from build123d import *

# Parameters (mm, degrees)
SKETCH1_W                   = 800
SKETCH1_H                   = 50
BOSS_EXTRUDE1_DEPTH         = 30
SKETCH2_R                   = 40
BOSS_EXTRUDE2_DEPTH         = 370
FILLET5_RADIUS              = 25
FILLET5_LENGTH              = 30
FILLET6_R                   = 25
FILLET5_OF_MIRROR3_2_RADIUS = 25
FILLET5_OF_MIRROR3_2_LENGTH = 30
FILLET6_OF_MIRROR3_R        = 25
CUT_EXTRUDE3_DEPTH          = 589.680979382
CUT_EXTRUDE3_DEPTH_BACK     = 589.680979382
SKETCH5_R                   = 10
SKETCH6_R                   = 10
CUT_EXTRUDE4_DEPTH          = 589.680979382


with BuildPart() as part:
    # Sketch1 → Boss-Extrude1 (new body)
    with BuildSketch(Plane.XY):
        Rectangle(SKETCH1_W, SKETCH1_H)
    boss_extrude1 = extrude(amount=BOSS_EXTRUDE1_DEPTH)

    # Sketch2 → Boss-Extrude2 (add)
    with BuildSketch(Plane.XY.offset(30)):
        with Locations(Location((-360.056615351, 0, 0), (0, 0, 176.951220784))):
            Circle(SKETCH2_R)
    extrude(amount=BOSS_EXTRUDE2_DEPTH)

    # Fillet5: full round fillet: the end face becomes a half cylinder, R = half its width
    fillet5_face = Plane((400, 0, 15), x_dir=(0, 0, -1), z_dir=(1, 0, 0))  # on the end face: x along it, z out of the body
    fillet5_slab = fillet5_face.offset(-FILLET5_RADIUS / 2) * Box(FILLET5_LENGTH, 2 * FILLET5_RADIUS, FILLET5_RADIUS, mode=Mode.PRIVATE)  # the body's end, R deep
    fillet5_round = Plane((375, 0, 15), x_dir=(1, 0, 0), z_dir=(0, 0, -1)) * Cylinder(FILLET5_RADIUS, FILLET5_LENGTH, mode=Mode.PRIVATE)  # its axis R under the face
    add(fillet5_slab - fillet5_round, mode=Mode.SUBTRACT)

    # Fillet6
    # the kernel refuses this fillet: 25 mm, written as the material it takes off along each edge
    with BuildSketch(Plane(origin=(-400, -25, -62.5), x_dir=(0, 1, 0), z_dir=(0, 0, 1)), Plane(origin=(-400, 25, -62.5), x_dir=(1, 0, 0), z_dir=(0, 0, 1))) as fillet6_piece_1:
        with BuildLine():
            CenterArc((FILLET6_R, -FILLET6_R), FILLET6_R, 90, 90)
            Line((0, -FILLET6_R), (0, 0))
            Line((0, 0), (FILLET6_R, 0))
        make_face()
    extrude(amount=92.5, mode=Mode.SUBTRACT)

    # Mirror3: Boss-Extrude1 across plane
    add(boss_extrude1.mirror(Plane.XY.offset(215)))

    # Fillet5 of Mirror3 2: full round fillet: the end face becomes a half cylinder, R = half its width
    fillet5_of_mirror3_2_face = Plane((400, 0, 415), x_dir=(0, 0, 1), z_dir=(1, 0, 0))  # on the end face: x along it, z out of the body
    fillet5_of_mirror3_2_slab = fillet5_of_mirror3_2_face.offset(-FILLET5_OF_MIRROR3_2_RADIUS / 2) * Box(FILLET5_OF_MIRROR3_2_LENGTH, 2 * FILLET5_OF_MIRROR3_2_RADIUS, FILLET5_OF_MIRROR3_2_RADIUS, mode=Mode.PRIVATE)  # the body's end, R deep
    fillet5_of_mirror3_2_round = Plane((375, 0, 415), x_dir=(1, 0, 0), z_dir=(0, 0, 1)) * Cylinder(FILLET5_OF_MIRROR3_2_RADIUS, FILLET5_OF_MIRROR3_2_LENGTH, mode=Mode.PRIVATE)  # its axis R under the face
    add(fillet5_of_mirror3_2_slab - fillet5_of_mirror3_2_round, mode=Mode.SUBTRACT)

    # Fillet6 of Mirror3
    # the kernel refuses this fillet: 25 mm, written as the material it takes off along each edge
    with BuildSketch(Plane(origin=(-400, -25, 492.5), x_dir=(0, 1, 0), z_dir=(0, 0, -1))) as fillet6_of_mirror3_piece_1:
        with BuildLine():
            CenterArc((FILLET6_OF_MIRROR3_R, FILLET6_OF_MIRROR3_R), FILLET6_OF_MIRROR3_R, 180, 90)
            Line((0, FILLET6_OF_MIRROR3_R), (0, 0))
            Line((0, 0), (FILLET6_OF_MIRROR3_R, 0))
        make_face()
    extrude(amount=92.5, mode=Mode.SUBTRACT)
    with BuildSketch(Plane(origin=(-400, 25, 492.5), x_dir=(0, -1, 0), z_dir=(0, 0, -1))) as fillet6_of_mirror3_piece_2:
        with BuildLine():
            CenterArc((FILLET6_OF_MIRROR3_R, -FILLET6_OF_MIRROR3_R), FILLET6_OF_MIRROR3_R, 90, 90)
            Line((0, -FILLET6_OF_MIRROR3_R), (0, 0))
            Line((0, 0), (FILLET6_OF_MIRROR3_R, 0))
        make_face()
    extrude(amount=92.5, mode=Mode.SUBTRACT)

    # Sketch5 → Cut-Extrude3 (cut, two sides: drawn at the far end of the back side and taken through both)
    with BuildSketch(Plane.XY.offset(430).offset(-CUT_EXTRUDE3_DEPTH_BACK)):
        with Locations(Location((75, 0, 0), (0, 0, 180))):
            Circle(SKETCH5_R)
    extrude(amount=CUT_EXTRUDE3_DEPTH + CUT_EXTRUDE3_DEPTH_BACK, mode=Mode.SUBTRACT)

    # Sketch6 → Cut-Extrude4 (cut, through all)
    with BuildSketch(Plane.XY.offset(430)):
        with Locations((375, 0)):
            Circle(SKETCH6_R)
    extrude(amount=-CUT_EXTRUDE4_DEPTH, mode=Mode.SUBTRACT)


solid = part.part
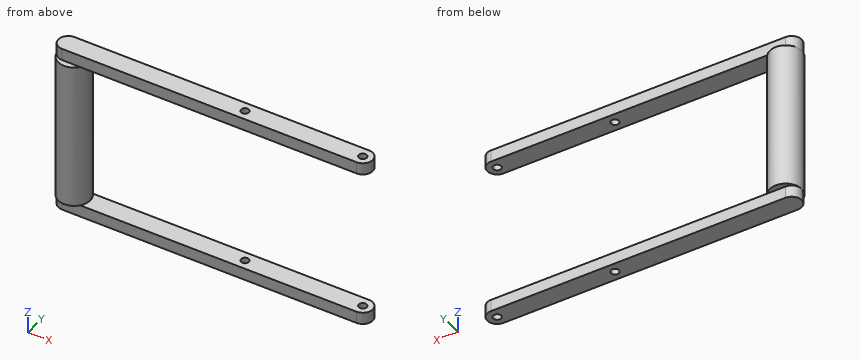
Read the model definition and answer for the solid it produces. Units are mm, in the model's axes. Round coordinates to 2 decimals unless told otherwise and drop trailing zeros. Order: outer loops, then holes, each group sorted by start corner. A loop starts at its lowest first (then second) coordinate and runs counter-clockwise, first axis right, second up.
1) The part is cut by section B-B on x = 75. Write down the section's boundary in (y, z).
2) Straight lines are drawn through the part: L1, parallel to Y at x = 375, z = 8.25; L2, parallel to Z at x = -133, y = 17; L3, parallel to X at y = -2.5, z = 378. For each, find the intervals that lie inside material, in ascending order.
3) The part is cut by section A-A on x = 179.5. Write down the section's boundary in (y, z), plus the area to 3 significant figures.
4) Flat-ended cylindrical pins translate along their axes: pin 1 (5 mm diameter, centred on y = -30.5, z = 168.5, fed in from +X); pin 2 (9 mm diameter, centred on x = -42.5, z = 21.5, fed in from -Y); pin 3 (3 mm diameter, centred on y = -30, z = 225.5, fed in from +X). Find the tip coordinate at first contact, or state that the pin passes through.
5) The part is cut by section C-C on z = 72.5. Write down the section's boundary in (x, y), plus the area to 3 significant figures.
Resolved:
1. outline: (-25, 0) - (-10, 0) - (-10, 30) - (-25, 30) - close; (-25, 400) - (-10, 400) - (-10, 430) - (-25, 430) - close; (10, 0) - (25, 0) - (25, 30) - (10, 30) - close; (10, 400) - (25, 400) - (25, 430) - (10, 430) - close
2. L1: y = -25 to -10, 10 to 25
2. L2: z = 0 to 30, 400 to 430
2. L3: x = -399.98 to -320.13
3. outline: (-25, 0) - (25, 0) - (25, 30) - (-25, 30) - close; (-25, 400) - (25, 400) - (25, 430) - (-25, 430) - close
3. area: 3,000 mm2
4. pin 1: stops at x = -331.49
4. pin 2: stops at y = -25
4. pin 3: stops at x = -331.99
5. outline: circle Ø80 at (-360.06, 0)
5. area: 5,030 mm2
